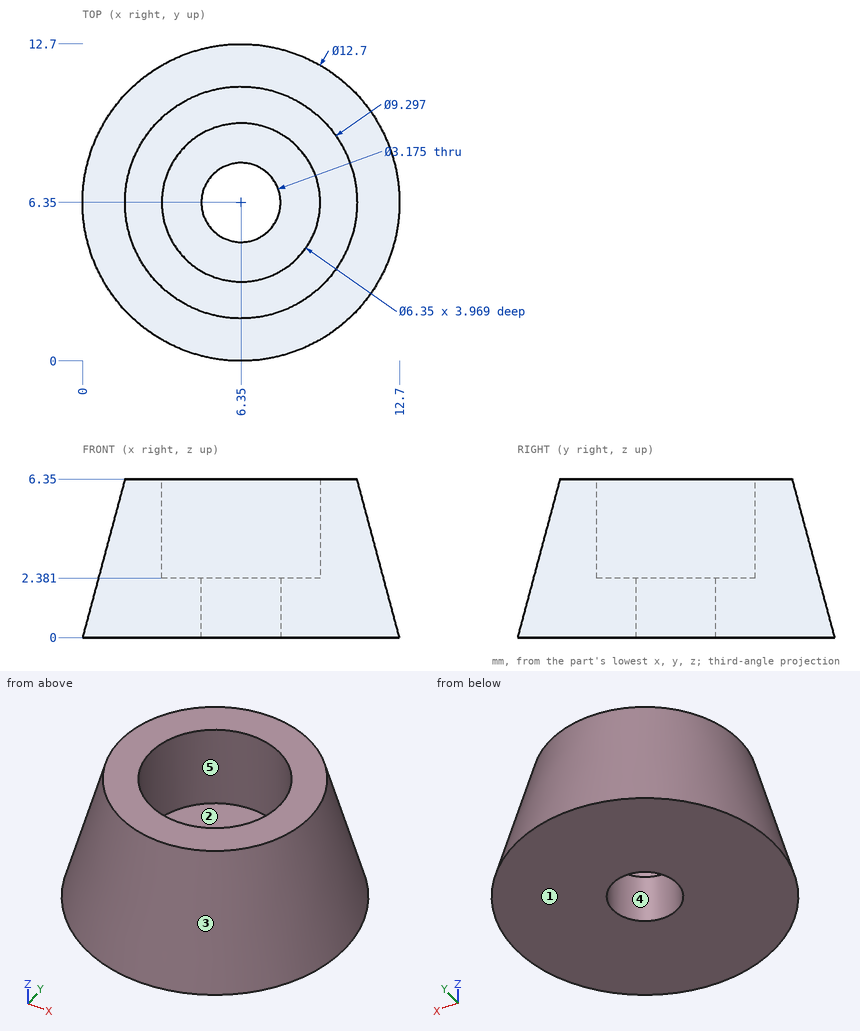
Part print with two shaded views. Sizes in mm from the minimum x, y, z corner. A direction names the side the tool comes from. Give positions to 0.01 mm unless a question says otherwise; leave off trailing zeros. Write each question's results on one line, items separated by ' | '.
1. 3-axis set-ups, long thin cutter, end or side, ignore diameter. For the marked faces 4 and 5: which of +Z, -Z, +X, -X, +Y, -Y reach the whole face in a straight line?
Calculated:
face 4: +Z, -Z | face 5: +Z
2. Pull direction Y, two halves, no side cores. Call the marked faces 1, 2 and 3: released by +Y, released by -Y, zero draft, split by the parting line, or undercut.
Calculated:
face 1: zero draft | face 2: undercut | face 3: split by the parting line
3. Pin check, flat tips, straight feed: pin 1 (1.9 mm diameter, centred on x = 6.35, y = 6.35, fed in from -Z); pin 2 (2 mm diameter, centred on y = 4.5, z = 3, fed in from -X); pin 3 (2 mm diameter, centred on y = 9, z = 1.5, fed in from -X). Stop position of each tip, or through.
Calculated:
pin 1: passes through | pin 2: stops at x = 0.73 | pin 3: stops at x = 0.53
4. Probe L1, parallel to Y at x = 8, z = 5.75; L2, parallel to X at y = 7.25, z = 1.75; L3, parallel to Y at x = 6.35, z = 0.9. List the from-to ranges inside material, lowest first. Write a range as from..to.
Calculated:
L1: y = 1.83..3.64, 9.06..10.87 | L2: x = 0.54..5.04, 7.66..12.16 | L3: y = 0.24..4.76, 7.94..12.46
